Input: part model. Units: mm. Frame: model coordinates. Face numbers are marked on the shaded views. Give positions to 0.01 mm unless a question says otherwise; leave off trailing zeros. Loops run counter-clockwise (first coordinate to the right, second up) from the corner with the lowest first, then second, coordinate; pieces in that order, holes last. Notation, with made-up numbers: (-21, 15.5) -> (17, 15.5) arc R25 ccw to (17, 51.5) -> close; hole circle Ø1 at (50.25, -29). An arc over 180 degrees is marked (long way). Answer in a Markdown table with one row per item. Add a question column.
```python
from build123d import *

# Parameters (mm, degrees)
SKETCH2_W           = 25
SKETCH2_H           = 168
BOSS_EXTRUDE1_DEPTH = 5
SKETCH3_W           = 10
SKETCH3_H           = 168
BOSS_EXTRUDE2_DEPTH = 5
SKETCH4_W           = 40
SKETCH4_H           = 25
BOSS_EXTRUDE3_DEPTH = 5
SKETCH5_W           = 25
SKETCH5_H           = 168
BOSS_EXTRUDE4_DEPTH = 5
SKETCH6_W           = 10
SKETCH6_H           = 168
BOSS_EXTRUDE5_DEPTH = 5
CUT_EXTRUDE1_DEPTH  = 5
CUT_EXTRUDE2_DEPTH  = 20
SKETCH9_W           = 2.75
SKETCH9_H           = 2.75
SKETCH9_H_2         = 2.689417066
CUT_EXTRUDE3_DEPTH  = 20
SKETCH10_W          = 2.75
SKETCH10_H          = 2.75
SKETCH10_H_2        = 3.15
CUT_EXTRUDE4_DEPTH  = 20
SKETCH11_W          = 2.75
SKETCH11_H          = 2.75
SKETCH11_W_2        = 2.782071424
SKETCH11_W_3        = 2.74
SKETCH11_H_2        = 2.74
CUT_EXTRUDE5_DEPTH  = 20
SKETCH12_W          = 2.75
SKETCH12_H          = 2.75
CUT_EXTRUDE6_DEPTH  = 20
SKETCH13_W          = 2.75
SKETCH13_H          = 2.75
SKETCH13_W_2        = 2.699527024
CUT_EXTRUDE7_DEPTH  = 20


with BuildPart() as part:
    # Sketch2 → Boss-Extrude1 (new body)
    with BuildSketch(Plane.XY):
        Rectangle(SKETCH2_W, SKETCH2_H)
    extrude(amount=BOSS_EXTRUDE1_DEPTH)

    # Sketch3 → Boss-Extrude2 (add)
    with BuildSketch(Plane.ZY.offset(12.5)):
        with Locations((-5, 0)):
            Rectangle(SKETCH3_W, SKETCH3_H)
    extrude(amount=-BOSS_EXTRUDE2_DEPTH)

    # Sketch4 → Boss-Extrude3 (add)
    with BuildSketch(Plane.XY.offset(5)):
        with Locations((32.5, 42)):
            Rectangle(SKETCH4_W, SKETCH4_H)
    extrude(amount=-BOSS_EXTRUDE3_DEPTH)

    # Sketch5 → Boss-Extrude4 (add)
    with BuildSketch(Plane.XY.offset(5)):
        with Locations((65, 0)):
            Rectangle(SKETCH5_W, SKETCH5_H)
    extrude(amount=-BOSS_EXTRUDE4_DEPTH)

    # Sketch6 → Boss-Extrude5 (add)
    with BuildSketch(Plane(origin=(77.5, 0, 0), x_dir=(0, 0, -1), z_dir=(1, 0, 0))):
        with Locations((5, 0)):
            Rectangle(SKETCH6_W, SKETCH6_H)
    extrude(amount=-BOSS_EXTRUDE5_DEPTH)

    # Sketch7 → Cut-Extrude1 (cut)
    with BuildSketch(Plane.XY.offset(5)):
        with BuildLine():
            Line((14.965887672, 53.5), (50.034112328, 53.5))
            ThreePointArc((50.034112328, 53.5), (51.409112328, 52.125), (50.034112328, 50.75))
            Line((50.034112328, 50.75), (14.965887672, 50.75))
            ThreePointArc((14.965887672, 50.75), (13.590887672, 52.125), (14.965887672, 53.5))
        make_face()
    extrude(amount=-CUT_EXTRUDE1_DEPTH, mode=Mode.SUBTRACT)

    # Sketch8 → Cut-Extrude2 (cut)
    with BuildSketch(Plane.XY.offset(5)):
        with BuildLine():
            Line((73.500571176, -65.375), (56.499428824, -65.375))
            ThreePointArc((56.499428824, -65.375), (55.124428824, -64), (56.499428824, -62.625))
            Line((56.499428824, -62.625), (73.500571176, -62.625))
            ThreePointArc((73.500571176, -62.625), (74.875571176, -64), (73.500571176, -65.375))
        make_face()
    extrude(amount=-CUT_EXTRUDE2_DEPTH, mode=Mode.SUBTRACT)

    # Sketch9 → Cut-Extrude3 (cut)
    with BuildSketch(Plane.XY.offset(5)):
        with Locations((6.35, 44.38125)):
            Rectangle(SKETCH9_W, SKETCH9_H)
        with Locations((-6.35, 44.38125)):
            Rectangle(SKETCH9_W, SKETCH9_H)
        with Locations((-6.35, 39.61875)):
            Rectangle(SKETCH9_W, SKETCH9_H_2)
        with Locations((6.35, 39.61875)):
            Rectangle(SKETCH9_W, SKETCH9_H_2)
    extrude(amount=-CUT_EXTRUDE3_DEPTH, mode=Mode.SUBTRACT)

    # Sketch10 → Cut-Extrude4 (cut)
    with BuildSketch(Plane.XY.offset(5)):
        with Locations((58.65, 50.63125)):
            Rectangle(SKETCH10_W, SKETCH10_H)
        with Locations((71.35, 50.63125)):
            Rectangle(SKETCH10_W, SKETCH10_H)
        with Locations((58.65, 45.86875)):
            Rectangle(SKETCH10_W, SKETCH10_H)
        with Locations((71.35, 45.86875)):
            Rectangle(SKETCH10_W, SKETCH10_H)
        with Locations((71.35, 38.13125)):
            Rectangle(SKETCH10_W, SKETCH10_H)
        with Locations((58.65, 38.13125)):
            Rectangle(SKETCH10_W, SKETCH10_H)
        with Locations((58.65, 33.36875)):
            Rectangle(SKETCH10_W, SKETCH10_H_2)
        with Locations((71.35, 33.36875)):
            Rectangle(SKETCH10_W, SKETCH10_H)
    extrude(amount=-CUT_EXTRUDE4_DEPTH, mode=Mode.SUBTRACT)

    # Sketch11 → Cut-Extrude5 (cut)
    with BuildSketch(Plane.XY.offset(5)):
        with Locations((58.65, -50.24375)):
            Rectangle(SKETCH11_W, SKETCH11_H)
        with Locations((71.35, -50.24375)):
            Rectangle(SKETCH11_W_2, SKETCH11_H)
        with Locations((71.35, -55.00625)):
            Rectangle(SKETCH11_W_3, SKETCH11_H_2)
        with Locations((58.65, -55.00625)):
            Rectangle(SKETCH11_W, SKETCH11_H_2)
        with Locations((-6.35, -50.24375)):
            Rectangle(SKETCH11_W, SKETCH11_H)
        with Locations((6.35, -50.24375)):
            Rectangle(SKETCH11_W, SKETCH11_H)
        with Locations((6.35, -55.00625)):
            Rectangle(SKETCH11_W, SKETCH11_H_2)
        with Locations((-6.35, -55.00625)):
            Rectangle(SKETCH11_W, SKETCH11_H_2)
    extrude(amount=-CUT_EXTRUDE5_DEPTH, mode=Mode.SUBTRACT)

    # Sketch12 → Cut-Extrude6 (cut)
    with BuildSketch(Plane.XY.offset(5)):
        with Locations((-3.175, -75.643809518)):
            Rectangle(SKETCH12_W, SKETCH12_H)
        with Locations((3.175, -75.643809518)):
            Rectangle(SKETCH12_W, SKETCH12_H)
        with Locations((3.175, -80.406309518)):
            Rectangle(SKETCH12_W, SKETCH12_H)
        with Locations((-3.175, -80.406309518)):
            Rectangle(SKETCH12_W, SKETCH12_H)
    extrude(amount=-CUT_EXTRUDE6_DEPTH, mode=Mode.SUBTRACT)

    # Sketch13 → Cut-Extrude7 (cut)
    with BuildSketch(Plane.XY.offset(5)):
        with Locations((-2.54, -41.237096808)):
            Rectangle(SKETCH13_W, SKETCH13_H)
        with Locations((2.54, -41.237096808)):
            Rectangle(SKETCH13_W, SKETCH13_H)
        with Locations((62.46, -41.237096808)):
            Rectangle(SKETCH13_W_2, SKETCH13_H)
        with Locations((67.54, -41.237096808)):
            Rectangle(SKETCH13_W, SKETCH13_H)
    extrude(amount=-CUT_EXTRUDE7_DEPTH, mode=Mode.SUBTRACT)


solid = part.part
```
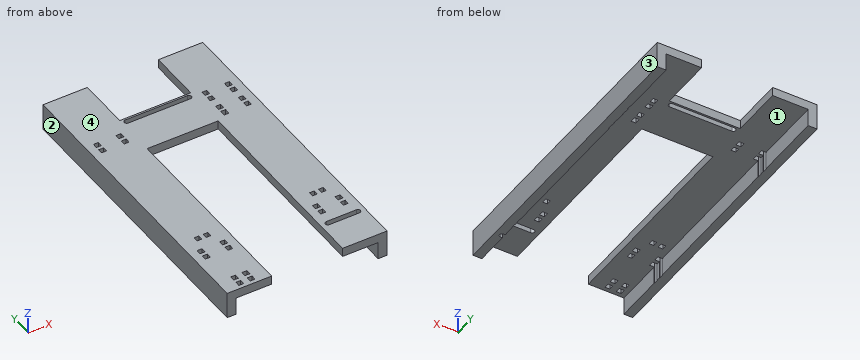
1) Section B-B on x = 38. Output: boundary loops of the cut face in (y, z).
2) Material intervals for line 1 along X through (y, z) = (24, -0.5); line 2 along X through (y, z) = (64.5, 4.25); line 3 along Y through (x, z) = (62.5, 1.75) (3 decimals), sorted ascending.
3) Section C-C on z = 2.5. State how many separate pieces and enclosed holes the cut face has, and give its area (3 significant figures).
4) Pull-direction query (X, two-part tool) for the marked faces 1, 2, 3 and 4; classes: +X half, -X half, draft (parallel to the pull), parting line (faces both ways), or undercut.
5) Section A-A on y = -26.5. Output: boundary loops of the cut face in (x, z).
6) Pin query (flat end, axial travel): pin 1 (12 mm diameter, centred on x = 44, y = 34.5, fed in from -Z); pin 2 (2.5 mm diameter, centred on x = 28, z = 3.5, fed in from +Y). Return the tip coordinate at first contact, or that it passes through.
Working result:
| question | item | result |
|---|---|---|
| 1 | outline | (29.5, 0) -> (50.75, 0) -> (50.75, 5) -> (29.5, 5) -> close; (53.5, 0) -> (54.5, 0) -> (54.5, 5) -> (53.5, 5) -> close |
| 2 | line 1 | x = -12.5 to -7.5, 72.5 to 77.5 |
| 2 | line 2 | x = -12.5 to 12.5, 52.5 to 77.5 |
| 2 | line 3 | y = -84 to -65.375, -62.625 to -42.612, -39.862 to 84 |
| 3 | separate pieces | 1 |
| 3 | enclosed holes | 30 |
| 3 | area | 9,030 mm2 |
| 4 | face 1 | undercut |
| 4 | face 2 | -X half |
| 4 | face 3 | +X half |
| 4 | face 4 | draft |
| 5 | outline | (-12.5, -10) -> (-7.5, -10) -> (-7.5, 0) -> (12.5, 0) -> (12.5, 5) -> (-12.5, 5) -> close; (52.5, 0) -> (72.5, 0) -> (72.5, -10) -> (77.5, -10) -> (77.5, 5) -> (52.5, 5) -> close |
| 6 | pin 1 | stops at z = 0 |
| 6 | pin 2 | stops at y = 54.5 |
